```python
from build123d import *

# Parameters (mm, degrees)
BOX027_W     = 70
BOX027_H     = 87
BOX027_DEPTH = 39
FILLET050_R  = 2
BOX031_W     = 74
BOX031_H     = 91
BOX031_DEPTH = 27
FILLET046_R  = 2


with BuildPart() as bottomcut013:
    # Box027 → Box027 (new body)
    with BuildSketch(Plane(origin=(2, 2, 2), x_dir=(1, 0, 0), z_dir=(0, 0, 1))):
        with Locations((35, 43.5)):
            Rectangle(BOX027_W, BOX027_H)
    extrude(amount=BOX027_DEPTH)

    # Fillet050
    fillet050_edges = [bottomcut013.edges().sort_by_distance(p)[0] for p in [
        (2, 2, 21.5),
        (2, 89, 21.5),
        (2, 45.5, 2),
        (72, 2, 21.5),
        (72, 89, 21.5),
        (72, 45.5, 2),
        (37, 2, 2),
        (37, 89, 2),
    ]]
    fillet(fillet050_edges, radius=FILLET050_R)


with BuildPart() as bottom052:
    # Box031 → Box031 (new body)
    with BuildSketch(Plane.XY):
        with Locations((37, 45.5)):
            Rectangle(BOX031_W, BOX031_H)
    extrude(amount=BOX031_DEPTH)

    # Fillet046
    fillet046_edges = [bottom052.edges().sort_by_distance(p)[0] for p in [
        (0, 0, 13.5),
        (0, 91, 13.5),
        (0, 45.5, 0),
        (74, 0, 13.5),
        (74, 91, 13.5),
        (74, 45.5, 0),
        (37, 0, 0),
        (37, 91, 0),
    ]]
    fillet(fillet046_edges, radius=FILLET046_R)

    # Cut032: cut bottomCut013
    add(bottomcut013.part, mode=Mode.SUBTRACT)


solid = bottom052.part
```
Design review of the part built by this model. Coordinates are the model's own, in mm. A direction names the side the tool comes from. Give positions to 0.01 mm unless a question says otherwise; leave off trailing zeros. Loops run counter-clockwise (first coordinate to the right, second up) from the corner with the lowest first, then second, coordinate; pieces in that order, holes last. Notation, with made-up numbers: M 37,-8.5 L 41,-8.5 A9 cw 41,5.5 Z; hole C -32.75,89.5 d5. An arc over 180 degrees is marked long. Return JSON: item names as keys, results as strings. Group by question number.
Item 1: Tool access review of faces 1 (the cylindrical face through (73.43, 90.4, 14.68)), 2 (the cylindrical face through (2.57, 46.08, 2.6)): name each direction out of +Z, -Z, +X, -X, +Y, -Y from which nothing blocks a thin tool from reaching the whole face with its end or side.
Item 2: Mouldability with a two-part tool opening along Y and no side actions: class faces 3 (the cylindrical face through (37.49, 0.57, 0.6)), 4 (the flat face through (1, 46, 27)), 5 (the flat face through (2, 45, 15)) as released by +Y, released by -Y, zero draft, split by the parting line, or undercut.
Item 3: Insertion check: pin 1 Ø2 at (x, y) = (46.5, 74) entering from +Z. The pin has a flat end and moves straight along its axis. Give the tip position at first contact, or say it passes through.
Item 4: For probe 1 along Y at (x, z) = (43, 23.75); probe 2 along X at (y, z) = (46.5, 8); probe 3 along Z at (x, y) = (14.5, 38), list the stretches that pass through material, from the lowest coordinate up.
Item 5: We need section A-A (x = 66.5). Give the boundary of the cut face in (y, z), and give its area (3 significant figures).
Item 6: We need section C-C (y = 59.5). Give the boundary of the cut face in (x, z).
Item 7: We need section B-B (z = 8.25). Give the boundary of the cut face in (x, y).
Item 8: We need section D-D (z = 3). Give the boundary of the cut face in (x, y), and give its area (3 significant figures).
Output:
{
 "1": {"face 1": "+Z, -Z, +X, +Y", "face 2": "+Z"},
 "2": {"face 3": "released by -Y", "face 4": "zero draft", "face 5": "undercut"},
 "3": {"pin 1": "stops at z = 2"},
 "4": {"probe 1": "y = 0 to 2, 89 to 91", "probe 2": "x = 0 to 2, 72 to 74", "probe 3": "z = 0 to 2"},
 "5": {"outline": "M 0,2 A2 ccw 2,0 L 89,0 A2 ccw 91,2 L 91,27 L 89,27 L 89,4 A2 cw 87,2 L 4,2 A2 cw 2,4 L 2,27 L 0,27 Z", "area": "282 mm^2"},
 "6": {"outline": "M 0,2 A2 ccw 2,0 L 72,0 A2 ccw 74,2 L 74,27 L 72,27 L 72,4 A2 cw 70,2 L 4,2 A2 cw 2,4 L 2,27 L 0,27 Z"},
 "7": {"outline": "M 0,2 A2 ccw 2,0 L 72,0 A2 ccw 74,2 L 74,89 A2 ccw 72,91 L 2,91 A2 ccw 0,89 Z; hole M 2,4 A2 ccw 4,2 L 70,2 A2 ccw 72,4 L 72,87 A2 ccw 70,89 L 4,89 A2 ccw 2,87 Z"},
 "8": {"outline": "M 0,2 A2 ccw 2,0 L 72,0 A2 ccw 74,2 L 74,89 A2 ccw 72,91 L 2,91 A2 ccw 0,89 Z; hole M 2.27,4 A1.73 ccw 4,2.27 L 70,2.27 A1.73 ccw 71.73,4 L 71.73,87 A1.73 ccw 70,88.73 L 4,88.73 A1.73 ccw 2.27,87 Z", "area": "727 mm^2"}
}
